Build history of the part. All positions in model axes, mm. Round coordinates to 2 decimals unless told otherwise and drop trailing zeros. Write each loop counter-clockwise with the first axis right and the second up, starting at its lowest first coordinate (ties: lowest second). Pieces come first, ordered by that corner, then holes. Notation, with made-up numbers: (55, 64.25) - (102, 64.25) arc R23 cw to (102, 99.25) - close; hole circle Ø8 at (-14.5, -31.75). An arc over 180 degrees is marked (long way). One line per question, with ' | ' between items.
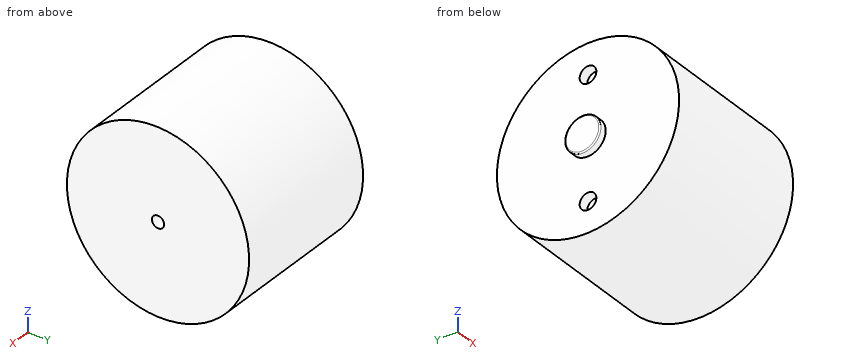
from build123d import *

# Parameters (mm, degrees)
SKETCH1_W           = 30
SKETCH1_H           = 18
SKETCH2_R           = 1.2
CUT_EXTRUDE1_DEPTH  = 4
SKETCH3_R           = 3.5
BOSS_EXTRUDE1_DEPTH = 1.5
FILLET1_R           = 0.25
SKETCH4_R           = 1.65
CUT_EXTRUDE2_DEPTH  = 2


with BuildPart() as part:
    # Sketch1 → Revolve1 (revolve)
    with BuildSketch(Plane.XY, mode=Mode.PRIVATE) as revolve1_sk:
        with Locations((-10, 9)):
            Rectangle(SKETCH1_W, SKETCH1_H)
    revolve(revolve1_sk.sketch.rotate(Axis((-25, 0, 0), (1, 0, 0)), 90), axis=Axis((-25, 0, 0), (1, 0, 0)))

    # Sketch2 → Cut-Extrude1 (cut)
    with BuildSketch(Plane(origin=(5, 0, 0), x_dir=(0, 0, -1), z_dir=(1, 0, 0))):
        Circle(SKETCH2_R)
    extrude(amount=-CUT_EXTRUDE1_DEPTH, mode=Mode.SUBTRACT)

    # Sketch3 → Boss-Extrude1 (add)
    with BuildSketch(Plane.ZY.offset(25)):
        Circle(SKETCH3_R)
    extrude(amount=BOSS_EXTRUDE1_DEPTH)

    # Fillet1
    fillet1_edges = [part.edges().sort_by_distance(p)[0] for p in [
        (-26.5, 0, -3.5),
    ]]
    fillet(fillet1_edges, radius=FILLET1_R)

    # Sketch4 → Cut-Extrude2 (cut)
    with BuildSketch(Plane.ZY.offset(25)):
        with Locations((-12, 0)):
            Circle(SKETCH4_R)
        with Locations((12, 0)):
            Circle(SKETCH4_R)
    extrude(amount=-CUT_EXTRUDE2_DEPTH, mode=Mode.SUBTRACT)


solid = part.part
Q1. Drop flat-ended pins along their axis: pin 1 (1.6 mm diameter, centred on y = 0.5, z = -12.5, fed in from -X); pin 2 (4.5 mm diameter, centred on y = 0, z = 12, fed in from -X); pin 3 (4 mm diameter, centred on x = -22, z = 14, fed in from +Y). Give the stop position or say it passes through.
Found:
pin 1: x = -23 | pin 2: x = -25 | pin 3: y = 13.42
Q2. Saw through at C-C, the plane x = -7.5. List the corners of the cut face in (y, z).
Found:
outline: circle Ø36 at (0, 0)
Q3. Saw through at D-D, the plane x = 3. List the corners of the cut face in (y, z), then the cut area to 3 significant figures.
Found:
outline: circle Ø36 at (0, 0); hole circle Ø2.4 at (0, 0) | area: 1,010 mm^2
Q4. Drill centre lines: L1, parallel to Y at x = 4, z = 0; L2, parallel to X at y = -6.5, z = 4; L3, parallel to Y at x = -24.25, z = -12. Where is each one in solid material? Low to high. Write a range as from..to.
Found:
L1: -18..-1.2, 1.2..18 | L2: -25..5 | L3: -13.42..-1.65, 1.65..13.42
Q5. Saw through at A-A, the plane y = 0. List the corners of the cut face in (x, z).
Found:
outline: (-26.5, -3.25) arc R0.25 ccw to (-26.25, -3.5) - (-25, -3.5) - (-25, -10.35) - (-23, -10.35) - (-23, -13.65) - (-25, -13.65) - (-25, -18) - (5, -18) - (5, -1.2) - (1, -1.2) - (1, 1.2) - (5, 1.2) - (5, 18) - (-25, 18) - (-25, 13.65) - (-23, 13.65) - (-23, 10.35) - (-25, 10.35) - (-25, 3.5) - (-26.25, 3.5) arc R0.25 ccw to (-26.5, 3.25) - close
Q6. Saw through at B-B, the plane z = 0. List the corners of the cut face in (x, y).
Found:
outline: (-26.5, -3.25) arc R0.25 ccw to (-26.25, -3.5) - (-25, -3.5) - (-25, -18) - (5, -18) - (5, -1.2) - (1, -1.2) - (1, 1.2) - (5, 1.2) - (5, 18) - (-25, 18) - (-25, 3.5) - (-26.25, 3.5) arc R0.25 ccw to (-26.5, 3.25) - close
